Autodesk Fusion 360 part; units mm, degrees
sketch "Sketch1" plane through (0, 0, 0) normal (0, 1, 0) x (1, 0, 0)
  line L0 (0, 0) -> (-20, 0)
  line L1 (-20, 0) -> (-20, 12)
  line L2 (-20, 12) -> (0, 12)
  line L3 (0, 12) -> (0, 0)
  dimension "d1" = 20
  dimension "d2" = 12
extrude "Extrude1" add sketch "Sketch1" along normal blind 2
sketch "Sketch2" plane through (0, 2, 0) normal (0, 1, 0) x (-1, 0, 0)
  line L0 (0, -12) -> (20, -12)
  line L1 (20, -12) -> (20, 0)
  line L2 (20, 0) -> (0, 0)
  line L3 (0, 0) -> (0, -12)
  circle A0 centre (10, -6) radius 5
  circle A1 centre (10, -6) radius 6
extrude "Extrude2" add sketch "Sketch2" along normal blind 5 contours A1
sketch "Sketch3" plane through (0, 0, 0) normal (0, 0, 1) x (1, 0, 0)
  line L0 (-20, 0) -> (0, 0)
  line L1 (0, 0) -> (0, 2)
  line L2 (0, 2) -> (-10, 2)
  line L3 (-10, 2) -> (-20, 2)
  line L4 (-20, 2) -> (-20, 0)
  line L5 (-17, 0) -> (-18, 0)
  line L6 (-18, 0) -> (-18, 1)
  line L7 (-18, 1) -> (-17, 1)
  line L8 (-17, 1) -> (-17, 0)
  line L9 (-2, 1) -> (-3, 1)
  line L10 (-3, 1) -> (-3, 0)
  line L11 (-3, 0) -> (-2, 0)
  line L12 (-2, 0) -> (-2, 1)
extrude "Extrude3" cut sketch "Sketch3" against normal blind 13 contours L0 L5 L6 L7 L8 | L0 L9 L10 L11 L12
sketch "Sketch4" plane through (0, 0, 0) normal (0, 0, 1) x (1, 0, 0)
  line L0 (-17, 1) -> (-17, 0)
  line L1 (-17, 0) -> (-3, 0)
  line L2 (-3, 0) -> (-3, 1)
  line L3 (-3, 1) -> (-2, 1)
  line L4 (-2, 1) -> (-2, 0)
  line L5 (-2, 0) -> (0, 0)
  line L6 (0, 0) -> (0, 2)
  line L7 (0, 2) -> (-10, 2)
  line L8 (-10, 2) -> (-20, 2)
  line L9 (-20, 2) -> (-20, 0)
  line L10 (-20, 0) -> (-18, 0)
  line L11 (-18, 0) -> (-18, 1)
  line L12 (-18, 1) -> (-17, 1)
sketch "Sketch5" plane through (0, 2, 0) normal (0, 1, 0) x (-1, 0, 0)
  circle A0 centre (10, -6) radius 5
  circle A1 centre (10, -6) radius 5
  circle A2 centre (10, -6) radius 4
extrude "Extrude4" add sketch "Sketch5" along normal blind 5
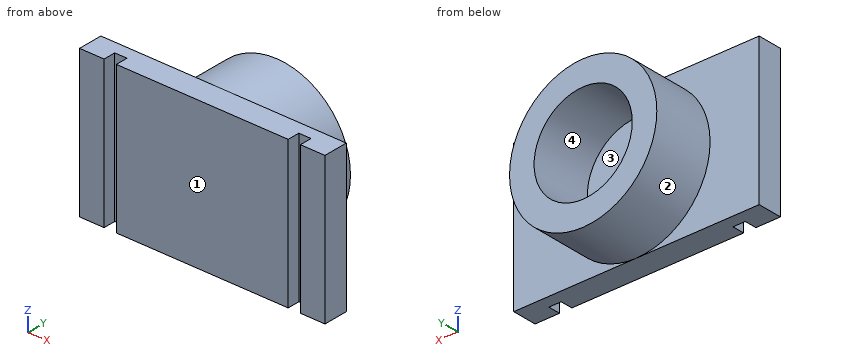
Check sheet for the modelled part. Datum: model origin and axes. Units: mm. Face numbers are marked on the shaded views. Coordinates: 2 decimals unless noted, no trailing zeros. Write each loop counter-clockwise with the first axis right and the second up, starting at its lowest first coordinate (ties: lowest second). Pieces come first, ordered by that corner, then holes. Notation, with made-up numbers: M -14.5,36.25 L 40.5,36.25 A34 ccw 40.5,67.25 Z; hole C -29,88.5 d3. An arc over 180 degrees is marked long. Write item = value, one per line. Start each with the question number.
1. Sectioned sample at A-A (z = -6). Record the cut outline in (x, y), then the cut area to 3 significant figures.
2. Sectioned sample at D-D (z = -9). Record the cut outline in (x, y).
3. Sectioned sample at C-C (x = -11). Record the cut outline in (y, z), then the cut area to 3 significant figures.
4. Mould release check, pull along X, two halves, no side actions. Record for the marked faces 1, 2, 3 and 4: pulls with the +X half, pulls with the -X half, needs draft (parallel to the pull), parting line crosses it, or undercut.
5. Sectioned sample at B-B (y = 4.75). Record the cut outline in (x, z).
6. Go/stop test with flat-tipped pins: pin 1 (1 mm diameter, centred on y = 4, z = -2.5, fed in from -X); pin 2 (0.5 mm diameter, centred on x = -2.5, z = -6.5, fed in from -Y); pin 3 (6.5 mm diameter, centred on x = -10, z = -6, fed in from +Y). Record where each tip stops, or that it passes through.
7. Thickness scan on probe 1 along Z at (x, y) = (-10, 5.95); probe 2 along Y at (x, z) = (-12, -3); probe 3 along Z at (x, y) = (-11.25, 6). Record the ranges inside material, lowest first.
The answers:
q1.outline = M -20,0 L -18,0 L -18,1 L -17,1 L -17,0 L -3,0 L -3,1 L -2,1 L -2,0 L 0,0 L 0,2 L -4,2 L -4,7 L -6,7 L -6,2 L -14,2 L -14,7 L -16,7 L -16,2 L -20,2 Z
q1.area = 58.0 mm²
q2.outline = M -20,0 L -18,0 L -18,1 L -17,1 L -17,0 L -3,0 L -3,1 L -2,1 L -2,0 L 0,0 L 0,2 L -4.8,2 L -4.8,7 L -7.35,7 L -7.35,2 L -12.65,2 L -12.65,7 L -15.2,7 L -15.2,2 L -20,2 Z
q3.outline = M 0,-12 L 2,-12 L 2,-11.92 L 7,-11.92 L 7,-9.87 L 2,-9.87 L 2,-2.13 L 7,-2.13 L 7,-0.08 L 2,-0.08 L 2,0 L 0,0 Z
q3.area = 44.4 mm²
q4.face_1 = needs draft
q4.face_2 = parting line crosses it
q4.face_3 = undercut
q4.face_4 = undercut
q5.outline = C -10,-6 d12; hole C -10,-6 d8
q6.pin_1 = -15.2
q6.pin_2 = 1
q6.pin_3 = 2
q7.probe_1 = -12 to -10, -2 to 0
q7.probe_2 = 0 to 2
q7.probe_3 = -11.87 to -9.8, -2.2 to -0.13
